```python
from build123d import *

# Parameters (mm, degrees)
SKETCH1_W           = 109.5
SKETCH1_H           = 83
SKETCH1_R           = 1.6
SKETCH1_R_2         = 1.3
BOSS_EXTRUDE1_DEPTH = 0.8
FILLET1_R           = 3
FILLET2_R           = 2


with BuildPart() as part:
    # Sketch1 → Boss-Extrude1 (new body)
    with BuildSketch(Plane.XY):
        with Locations((0, -41.5)):
            Rectangle(SKETCH1_W, SKETCH1_H)
        with Locations((23.55, -67.375)):
            Circle(SKETCH1_R, mode=Mode.SUBTRACT)
        with Locations((23.55, -15.625)):
            Circle(SKETCH1_R, mode=Mode.SUBTRACT)
        with Locations((48.25, -3.5)):
            Circle(SKETCH1_R, mode=Mode.SUBTRACT)
        with Locations((48.25, -79.5)):
            Circle(SKETCH1_R, mode=Mode.SUBTRACT)
        with Locations((-48.25, -79.5)):
            Circle(SKETCH1_R, mode=Mode.SUBTRACT)
        with Locations((-48.25, -3.5)):
            Circle(SKETCH1_R, mode=Mode.SUBTRACT)
        with Locations((-33.65, -2.07)):
            Circle(SKETCH1_R_2, mode=Mode.SUBTRACT)
        with Locations((-33.65, -11.6)):
            Circle(SKETCH1_R_2, mode=Mode.SUBTRACT)
        with Locations((39.75, -41.5)):
            Circle(SKETCH1_R, mode=Mode.SUBTRACT)
        Polygon((-50.25, -41.5), (-50.25, -61.5), (-44.75, -61.5), (-44.75, -79), (16.75, -79), (16.75, -64.5), (32.35, -64.5), (32.35, -18.5), (16.75, -18.5), (16.75, -4), (-28.25, -4), (-28.25, -16.1), (-44.75, -16.1), (-44.75, -21.5), (-50.25, -21.5), align=None, mode=Mode.SUBTRACT)
    extrude(amount=BOSS_EXTRUDE1_DEPTH)

    # Fillet1
    fillet1_edges = [part.edges().sort_by_distance(p)[0] for p in [
        (32.35, -64.5, 0.4),
        (32.35, -18.5, 0.4),
        (16.75, -18.5, 0.4),
        (16.75, -4, 0.4),
        (-28.25, -4, 0.4),
        (-28.25, -16.1, 0.4),
        (-44.75, -16.1, 0.4),
        (-50.25, -21.5, 0.4),
        (-50.25, -61.5, 0.4),
        (-44.75, -79, 0.4),
        (16.75, -79, 0.4),
        (16.75, -64.5, 0.4),
    ]]
    fillet(fillet1_edges, radius=FILLET1_R)

    # Fillet2
    fillet2_edges = [part.edges().sort_by_distance(p)[0] for p in [
        (-44.75, -21.5, 0.4),
        (-44.75, -61.5, 0.4),
    ]]
    fillet(fillet2_edges, radius=FILLET2_R)


solid = part.part
```
Geometry: final body of the model. Coordinates: model frame, mm. A direction names the side the tool comes from. Round coordinates to 2 decimals unless told otherwise and drop trailing zeros. Write each loop counter-clockwise with the first axis right and the second up, starting at its lowest first coordinate (ties: lowest second). Pieces come first, ordered by that corner, then holes. Notation, with made-up numbers: M 62.5,2 L 101.5,2 A29 cw 101.5,36 Z; hole C 11.25,-19.5 d9. An arc over 180 degrees is marked long. Answer in a Markdown table with one row per item. Add a question column.
(1) Draft query along X for faces 1 (the face through (36, -35, 0)), 2 (the face through (-27.39, -4.9, 0.41)). Return one class per face: pulls with the +X half, pulls with the -X half, needs draft (parallel to the pull), parting line crosses it, or undercut.
(2) Cut plane D-D, the plane y = -11.6. Return the cut outline in (x, z), then the cut area to 3 significant figures.
(3) Ray query, L1, parallel to X at y = -79.5, z = 0.45; L2, parallel to X at y = -46, z = 0.2; L3, parallel to Y at x = -39.5, z = 0.5. Return the intervals inside material, ascending.
(4) Cut plane C-C, the plane x = 39.75. Return the cut outline in (y, z).
(5) Contact query for a flat-ended pin moving along its axis: pin 1 (1.6 mm diameter, centred on x = -33.65, y = -2.07, fed in from -Z). Output: stop coordinate, or through.
(6) Cut plane A-A, the plane x = 23.55. Return the cut outline in (y, z) (3 decimals), then the cut area to 3 significant figures.
(7) Reachability of faces 3 (the face through (36, -35, 0.8)), 4 (the face through (-49.39, -22.4, 0.41)) from +Z, -Z, +X, -X, +Y, -Y: full face, straight path, thin tool, end or side. Return the list, or none.
(8) Cut plane B-B, the plane y = -33. Return the cut outline in (x, z), then the cut area to 3 significant figures.
Established:
| question | item | result |
|---|---|---|
| 1 | face 1 | needs draft |
| 1 | face 2 | undercut |
| 2 | outline | M -54.75,0 L -34.95,0 L -34.95,0.8 L -54.75,0.8 Z; M -32.35,0 L -28.25,0 L -28.25,0.8 L -32.35,0.8 Z; M 16.75,0 L 54.75,0 L 54.75,0.8 L 16.75,0.8 Z |
| 2 | area | 49.5 mm² |
| 3 | L1 | -54.75 to -49.85, -46.65 to 46.65, 49.85 to 54.75 |
| 3 | L2 | -54.75 to -50.25, 32.35 to 54.75 |
| 3 | L3 | -83 to -79, -16.1 to 0 |
| 4 | outline | M -83,0 L -43.1,0 L -43.1,0.8 L -83,0.8 Z; M -39.9,0 L 0,0 L 0,0.8 L -39.9,0.8 Z |
| 5 | pin 1 | through |
| 6 | outline | M -83,0 L -68.975,0 L -68.975,0.8 L -83,0.8 Z; M -65.775,0 L -64.5,0 L -64.5,0.8 L -65.775,0.8 Z; M -18.5,0 L -17.225,0 L -17.225,0.8 L -18.5,0.8 Z; M -14.025,0 L 0,0 L 0,0.8 L -14.025,0.8 Z |
| 6 | area | 24.5 mm² |
| 7 | face 3 | +Z, +X, -X, +Y, -Y |
| 7 | face 4 | +Z, -Z |
| 8 | outline | M -54.75,0 L -50.25,0 L -50.25,0.8 L -54.75,0.8 Z; M 32.35,0 L 54.75,0 L 54.75,0.8 L 32.35,0.8 Z |
| 8 | area | 21.5 mm² |
